Solid Edge part; units mm, degrees
sketch "Sketch1" plane through (0, 0, 0) normal (0, 0, 1) x (1, 0, 0)
  line L0 (92.5, 185) -> (-92.5, 185)
  line L1 (-92.5, 185) -> (-92.5, -185)
  line L2 (-92.5, -185) -> (92.5, -185)
  line L3 (92.5, -185) -> (92.5, 185)
  dimension "D1" = 92.5
  dimension "D2" = 92.5
extrude "Protrusion1" add sketch "Sketch1" along normal blind 400
sketch "Sketch2" plane through (-92.5, 0, 200) normal (-1, 0, 0) x (0, 0, 1)
  line L0 (190, -175) -> (-200, -175)
  line L1 (-200, -175) -> (-200, 175)
  line L2 (-200, 175) -> (190, 175)
  line L3 (190, 175) -> (190, -175)
  dimension "D1" = 200
extrude "ScavoEstrusione_2" cut sketch "Sketch2" against normal blind 175
fillet "Rotondo_1" radius 20 10 edges at (-5, 175, 390) (82.5, 0, 390) (-5, -175, 390) (82.5, -175, 195) (82.5, 175, 195) (92.5, 185, 200) (0, 185, 400) (92.5, 0, 400) (92.5, -185, 200) (0, -185, 400)
sketch "Sketch3" plane through (-10, -185, 190) normal (0, -1, 0) x (1, 0, 0)
  circle A0 centre (-47.5, -125) radius 5
  circle A1 centre (-17.5, -155) radius 5
  dimension "D1" = 47.5
extrude "Cutout1" cut sketch "Sketch3" against normal through all
properties material "Fe 360 B UNI 7070"
Read the model definition and answer for the solid it produces. Units are mm, in the model's axes. A direction names the side the tool comes from. Coordinates: 2 decimals unless noted, no trailing zeros. Order: outer loops, then holes, each group sorted by start corner. A loop starts at its lowest first (then second) coordinate and runs counter-clockwise, first axis right, second up. Notation, with made-up numbers: (47, -11.5) -> (74, -11.5) arc R19 cw to (74, -2.5) -> close; hole circle Ø10 at (-21, 82.25). An arc over 180 degrees is marked (long way). Answer as a JSON object with one key per item and string values.
1) A cutting plane is placed at C-C, the plane x = 28. Determine the outline of the cut face in (y, z), plus the area to 3 significant figures.
Model answer:
{"outline": "(-185, 0) -> (-175, 0) -> (-175, 370) arc R20 cw to (-155, 390) -> (155, 390) arc R20 cw to (175, 370) -> (175, 0) -> (185, 0) -> (185, 380) arc R20 ccw to (165, 400) -> (-165, 400) arc R20 ccw to (-185, 380) -> close", "area": "11,500 mm²"}
2) A tool of negligible diameter and unlimited length cuts with its end or side. For faces 1 (the face through (-11, -185, 187)), 2 (the face through (-16, 2, 390)), from which of +Z, -Z, +X, -X, +Y, -Y can it reach the whole face along a straight path? Write none if from no direction.
Model answer:
{"face 1": "+Z, -Z, +X, -X, -Y", "face 2": "-Z, -X"}
3) A cutting plane is placed at B-B, the plane x = -57.5. Determine the outline of the cut face in (y, z).
Model answer:
{"outline": "(-185, 0) -> (-175, 0) -> (-175, 60) -> (-185, 60) -> close; (-185, 70) -> (-175, 70) -> (-175, 370) arc R20 cw to (-155, 390) -> (155, 390) arc R20 cw to (175, 370) -> (175, 70) -> (185, 70) -> (185, 380) arc R20 ccw to (165, 400) -> (-165, 400) arc R20 ccw to (-185, 380) -> close; (175, 0) -> (185, 0) -> (185, 60) -> (175, 60) -> close"}
4) The mould has two halves that part along Y. Classify faces 3 (the face through (82.5, -2, 182)), 4 (the face through (-61.185, 179.93, 68.379)), 5 (the face through (86.486, -179.297, 192.66)): released by +Y, released by -Y, zero draft, split by the parting line, or undercut.
Model answer:
{"face 3": "undercut", "face 4": "zero draft", "face 5": "released by -Y"}
5) A cutting plane is placed at A-A, the plane z = 35. Determine the outline of the cut face in (x, y), plus the area to 3 significant figures.
Model answer:
{"outline": "(-92.5, -185) -> (-32.5, -185) -> (-32.5, -175) -> (-92.5, -175) -> close; (-92.5, 175) -> (-32.5, 175) -> (-32.5, 185) -> (-92.5, 185) -> close; (-22.5, -185) -> (72.5, -185) arc R20 ccw to (92.5, -165) -> (92.5, 165) arc R20 ccw to (72.5, 185) -> (-22.5, 185) -> (-22.5, 175) -> (62.5, 175) arc R20 cw to (82.5, 155) -> (82.5, -155) arc R20 cw to (62.5, -175) -> (-22.5, -175) -> close", "area": "7,000 mm²"}
6) Each of these flat-tipped pins is pushed along its axis until it touches: pin 1 (6 mm diameter, centred on x = -27.5, z = 35, fed in from -Y); pin 2 (8 mm diameter, centred on y = 81, z = 313.5, fed in from -X); pin 3 (1.5 mm diameter, centred on x = 48.5, y = -50, fed in from -Z); pin 4 (11.5 mm diameter, centred on x = -57.5, z = 65, fed in from +Y). Where does it stop, or does it pass through?
Model answer:
{"pin 1": "passes through", "pin 2": "stops at x = 82.5", "pin 3": "stops at z = 390", "pin 4": "stops at y = 185"}
7) Consider line 1 along Y through (x, z) = (-37.5, 131); line 2 along Z through (x, y) = (2.5, -44); line 3 along Z through (x, y) = (-27.5, -178.25). Determine where each line is inside the solid, lowest interval first. Write a range as from..to.
Model answer:
{"line 1": "y = -185..-175, 175..185", "line 2": "z = 390..400", "line 3": "z = 0..30, 40..394.98"}
8) A cutting plane is placed at D-D, the plane y = -142. Determine the outline of the cut face in (x, z).
Model answer:
{"outline": "(-92.5, 390) -> (62.5, 390) arc R20 cw to (82.5, 370) -> (82.5, 0) -> (92.5, 0) -> (92.5, 380) arc R20 ccw to (72.5, 400) -> (-92.5, 400) -> close"}
